Source: CAD feature listing. Evaluate the final solid. Frame: model axes, mm. A direction names the side the tool comes from. Coordinates: 2 decimals unless noted, no trailing zeros. Order: outer loops, then holes, each group sorted by start corner. A loop starts at its lowest first (then second) coordinate and runs counter-clockwise, first axis right, second up.
Autodesk Fusion 360 part; units mm, degrees
sketch "Sketch1" plane through (0, 0, 0) normal (0, 0, 1) x (1, 0, 0)
  circle A0 centre (0, 0) radius 12.5
extrude "Extrude1" add sketch "Sketch1" along normal blind 2
sketch "Sketch2" plane through (0, 0, 2) normal (0, 0, 1) x (-1, 0, 0)
  circle A0 centre (0, 0) radius 12.5
  circle A1 centre (0, 0) radius 3
extrude "Extrude2" add sketch "Sketch2" along normal blind 10 contours A1
sketch "Sketch3" plane through (0, 0, 12) normal (0, 0, 1) x (-1, 0, 0)
  circle A0 centre (0, 0) radius 3
  circle A1 centre (0, 0) radius 3.25
  dimension "d8" = 6.5
extrude "Extrude3" add sketch "Sketch3" along normal blind 5 contours A0 | A1
chamfer "Chamfer1" distance 2.5 angle 45 1 edges at (3.0301, 1.1753, 17)
chamfer "Chamfer2" distance 0.25 angle 45 1 edges at (2.797, 1.0848, 12)
fillet "Fillet1" radius 1 1 edges at (2.797, -1.0848, 2)
1. Section query C-C on z = 14. Return loops of the section in (x, y), plus the area to 3 significant figures.
Findings:
outline: circle Ø6.5 at (0, 0)
area: 33.2 mm2
2. Access query for faces 4 (the face through (11.923, -3.755, 0.986)), 5 (the face through (2.579, -1.978, 13.232)). Directions: +Z, -Z, +X, -X, +Y, -Y. A direction counts if a zero-diameter tool reaches every point of the face in a straight line with its end or side. Return the directions, or none.
Findings:
face 4: +Z, -Z
face 5: +Z
3. Section query D-D on x = -8.25. Return loops of the section in (y, z).
Findings:
outline: (-9.39, 0) - (9.39, 0) - (9.39, 2) - (-9.39, 2) - close
4. Pin query (flat end, axial travel): P1, Ø4, axis at x = 0.5, z = 9, coming from the -Y side; P2, Ø10, axis at x = -8.5, z = 9, coming from the -Y side; P3, Ø3, axis at y = 4, z = 7.5, coming from the +X side; P4, Ø12, axis at x = -6, y = -8, coming from the +Z side. Return the tip coordinate at first contact, or that it passes through.
Findings:
P1: stops at y = -3
P2: passes through
P3: stops at x = 1.66
P4: stops at z = 2
5. Draft query along Z for faces 1 (the face through (3, 0, 7)), 2 (the face through (0.196, -0.885, 16.844)), 3 (the face through (0, 0, 0)). Return one class per face: released by +Z, released by -Z, zero draft, split by the parting line, or undercut.
Findings:
face 1: undercut
face 2: released by +Z
face 3: released by -Z
6. Ray query, line 1 (Z direction, x = -4.5, y = -7.75); line 2 (Y direction, x = 1, z = 16.25); line 3 (X direction, y = -5, z = 1.5). Return the intervals inside material, ascending.
Findings:
line 1: z = 0 to 2
line 2: y = -1.12 to 1.12
line 3: x = -11.46 to 11.46
